Can you work these out from the model? Positions are in its coordinate system, mm. Face numbers are marked on the shaded views. Round coordinates to 2 decimals unless told otherwise and drop trailing zeros. Loops run counter-clockwise (first coordinate to the right, second up) from the corner with the lowest first, then second, coordinate; pieces in that order, holes last.
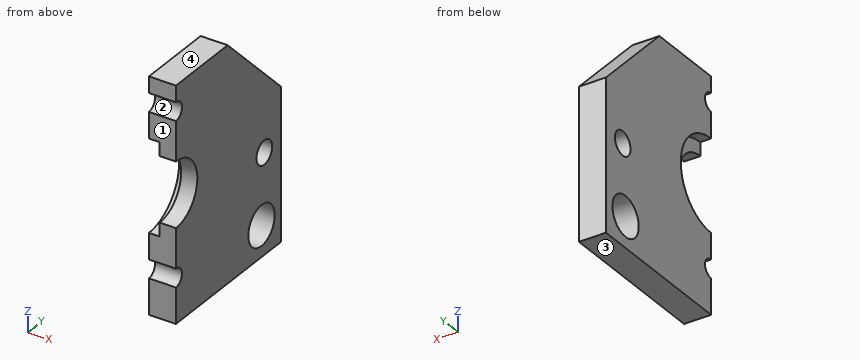
from build123d import *
from build123d import SkipClean  # not in build123d's __all__

# Parameters (mm, degrees)
F0_R     = 3.7
F0_R_2   = 2.2
F1_DEPTH = 5
F2_DEPTH = 3
F3_DEPTH = 5.001
F4_DEPTH = 2
F5_DEPTH = 2


# Not quite as in the source:
# - after a boolean that leaves OpenCascade's solid faulty, fix() repairs it
# - a feature names something its author has since deleted; it is built from what else it names


with BuildPart() as f1:
    # F0 (on Right) → F1 (new body)
    with BuildSketch(Plane.YZ):
        with BuildLine():
            Line((-33.3704365752, 11.9448962937), (-33.3704365752, 5.3711892086))
            Line((-33.3704365752, 5.3711892086), (-3.8608338702, 5.3711892086))
            Line((-3.8608338702, 5.3711892086), (-3.8608338702, 33.3448962937))
            Line((-3.8608338702, 33.3448962937), (-18.8608338702, 48.3448962937))
            Line((-18.8608338702, 48.3448962937), (-33.3704365752, 48.3448962937))
            Line((-33.3704365752, 48.3448962937), (-33.3704365752, 45.3448962937))
            ThreePointArc((-33.3704365752, 45.3448962937), (-31.6704365752, 43.6448962937), (-33.3704365752, 41.9448962937))
            Line((-33.3704365752, 41.9448962937), (-33.3704365752, 37.1448962937))
            ThreePointArc((-33.3704365752, 37.1448962937), (-24.8704365752, 28.6448962937), (-33.3704365752, 20.1448962937))
            Line((-33.3704365752, 20.1448962937), (-33.3704365752, 15.3448962937))
            ThreePointArc((-33.3704365752, 15.3448962937), (-31.6704365752, 13.6448962937), (-33.3704365752, 11.9448962937))
        make_face()
        with Locations((-9.3608338702, 11.0711892086)):
            Circle(F0_R, mode=Mode.SUBTRACT)
        with Locations((-8.5704365752, 23.8448962937)):
            Circle(F0_R_2, mode=Mode.SUBTRACT)
    extrude(amount=F1_DEPTH)

    # F0 (on Right) → F2 (join)
    with BuildSketch(Plane.YZ):
        with BuildLine():
            Line((-33.3704365752, 11.9448962937), (-33.3704365752, 5.3711892086))
            Line((-33.3704365752, 5.3711892086), (-3.8608338702, 5.3711892086))
            Line((-3.8608338702, 5.3711892086), (-3.8608338702, 33.3448962937))
            Line((-3.8608338702, 33.3448962937), (-18.8608338702, 48.3448962937))
            Line((-18.8608338702, 48.3448962937), (-33.3704365752, 48.3448962937))
            Line((-33.3704365752, 48.3448962937), (-33.3704365752, 45.3448962937))
            ThreePointArc((-33.3704365752, 45.3448962937), (-31.6704365752, 43.6448962937), (-33.3704365752, 41.9448962937))
            Line((-33.3704365752, 41.9448962937), (-33.3704365752, 37.1448962937))
            ThreePointArc((-33.3704365752, 37.1448962937), (-24.8704365752, 28.6448962937), (-33.3704365752, 20.1448962937))
            Line((-33.3704365752, 20.1448962937), (-33.3704365752, 15.3448962937))
            ThreePointArc((-33.3704365752, 15.3448962937), (-31.6704365752, 13.6448962937), (-33.3704365752, 11.9448962937))
        make_face()
        with Locations((-9.3608338702, 11.0711892086)):
            Circle(F0_R, mode=Mode.SUBTRACT)
        with Locations((-8.5704365752, 23.8448962937)):
            Circle(F0_R_2, mode=Mode.SUBTRACT)
        with BuildLine():
            Line((-33.3704365752, 15.3448962937), (-33.3704365752, 11.9448962937))
            ThreePointArc((-33.3704365752, 11.9448962937), (-31.6704365752, 13.6448962937), (-33.3704365752, 15.3448962937))
        make_face()
        with BuildLine():
            Line((-33.3704365752, 22.6448962937), (-33.3704365752, 20.1448962937))
            ThreePointArc((-33.3704365752, 20.1448962937), (-24.8704365752, 28.6448962937), (-33.3704365752, 37.1448962937))
            Line((-33.3704365752, 37.1448962937), (-33.3704365752, 34.6448962937))
            ThreePointArc((-33.3704365752, 34.6448962937), (-27.3704365752, 28.6448962937), (-33.3704365752, 22.6448962937))
        make_face()
        with BuildLine():
            Line((-33.3704365752, 34.6448962937), (-33.3704365752, 22.6448962937))
            ThreePointArc((-33.3704365752, 22.6448962937), (-27.3704365752, 28.6448962937), (-33.3704365752, 34.6448962937))
        make_face()
        with BuildLine():
            ThreePointArc((-33.3704365752, 41.9448962937), (-31.6704365752, 43.6448962937), (-33.3704365752, 45.3448962937))
            Line((-33.3704365752, 45.3448962937), (-33.3704365752, 41.9448962937))
        make_face()
    extrude(amount=F2_DEPTH)

    # F0 (on Right) → F3 (cut, through all)
    with BuildSketch(Plane.YZ):
        with BuildLine():
            Line((-33.3704365752, 34.6448962937), (-33.3704365752, 22.6448962937))
            ThreePointArc((-33.3704365752, 22.6448962937), (-27.3704365752, 28.6448962937), (-33.3704365752, 34.6448962937))
        make_face()
        with BuildLine():
            ThreePointArc((-33.3704365752, 41.9448962937), (-31.6704365752, 43.6448962937), (-33.3704365752, 45.3448962937))
            Line((-33.3704365752, 45.3448962937), (-33.3704365752, 41.9448962937))
        make_face()
        with BuildLine():
            Line((-33.3704365752, 15.3448962937), (-33.3704365752, 11.9448962937))
            ThreePointArc((-33.3704365752, 11.9448962937), (-31.6704365752, 13.6448962937), (-33.3704365752, 15.3448962937))
        make_face()
    with SkipClean():  # cleaning this boolean's faces spoils the solid; the shape is the same uncleaned
        extrude(amount=F3_DEPTH, mode=Mode.SUBTRACT)

    # F4 (add, through all): a face of the model
    f4_faces = [f1.faces().sort_by_distance(p)[0] for p in [
        (3, -25.0605023533, 28.6448962937),
    ]]
    extrude(f4_faces, amount=F4_DEPTH)

    add(f1.part.fix(), mode=Mode.REPLACE)

    # F0 (on Right) → F5 (cut)
    with BuildSketch(Plane.YZ):
        with BuildLine():
            Line((-33.3704365752, 22.6448962937), (-33.3704365752, 20.1448962937))
            ThreePointArc((-33.3704365752, 20.1448962937), (-24.8704365752, 28.6448962937), (-33.3704365752, 37.1448962937))
            Line((-33.3704365752, 37.1448962937), (-33.3704365752, 34.6448962937))
            ThreePointArc((-33.3704365752, 34.6448962937), (-27.3704365752, 28.6448962937), (-33.3704365752, 22.6448962937))
        make_face()
    extrude(amount=F5_DEPTH, mode=Mode.SUBTRACT)


solid = f1.part
(1) If we section it at B-B, the plane z = 11.5: List the corners of the cut face in (x, y) for me, then the cut area to 3 significant figures.
Worked answers:
outline: (0, -33.37) - (5, -33.37) - (5, -13.04) - (0, -13.04) - close; (0, -5.69) - (5, -5.69) - (5, -3.86) - (0, -3.86) - close
area: 111 mm2
(2) If we section it at A-A, the plane x = 1.4: List the corners of the cut face in (y, z) for me.
Worked answers:
outline: (-33.37, 5.37) - (-3.86, 5.37) - (-3.86, 33.34) - (-18.86, 48.34) - (-33.37, 48.34) - (-33.37, 45.34) arc R1.7 cw to (-33.37, 41.94) - (-33.37, 37.14) arc R8.5 cw to (-33.37, 20.14) - (-33.37, 15.34) arc R1.7 cw to (-33.37, 11.94) - close; hole circle Ø7.4 at (-9.36, 11.07); hole circle Ø4.4 at (-8.57, 23.84)
(3) If I drill on line 1 (Z direction, x = 3.3, y = -8); line 2 (Z direction, x = 0.4, y = -8.5); line 3 (Y direction, x = 1.1, z = 8), over which ranges is the centre line in solid material (lowest first)?
Worked answers:
line 1: z = 5.37 to 7.63, 14.51 to 21.72, 25.97 to 37.48
line 2: z = 5.37 to 7.47, 14.67 to 21.65, 26.04 to 37.98
line 3: y = -33.37 to -11.42, -7.3 to -3.86
(4) If we section it at D-D, the plane y = -26.25: List the corners of the cut face in (x, z) for me, then the cut area to 3 significant figures.
Worked answers:
outline: (0, 5.37) - (5, 5.37) - (5, 48.34) - (0, 48.34) - (0, 33.29) - (2, 33.29) - (2, 24) - (0, 24) - close
area: 196 mm2
(5) If we section it at C-C, the plane y = -30.25: List the corners of the cut face in (x, z) for me, then the cut area to 3 significant figures.
Worked answers:
outline: (0, 5.37) - (5, 5.37) - (5, 23.52) - (2, 23.52) - (2, 20.74) - (0, 20.74) - close; (0, 36.55) - (2, 36.55) - (2, 33.77) - (5, 33.77) - (5, 48.34) - (0, 48.34) - close
area: 152 mm2
(6) If we mould it in two halves opening along Z, with no side actions, what happens to the marked faces 1, 2, 3 and 4? For each: released by +Z, released by -Z, zero draft, split by the parting line, or undercut.
Worked answers:
face 1: zero draft
face 2: undercut
face 3: released by -Z
face 4: released by +Z
